Autodesk Inventor part; units mm, degrees
ref_plane "YZ Plane" through (0, 0, 0) normal (1, 0, 0) x (0, 1, 0)
ref_plane "XZ Plane" through (0, 0, 0) normal (0, 1, 0) x (-1, 0, 0)
ref_plane "XY Plane" through (0, 0, 0) normal (0, 0, 1) x (1, 0, 0)
sketch "スケッチ1" plane through (0, 0, 0) normal (0, 0, 1) x (1, 0, 0)
  line L0 (-22.9, 20) -> (-3.9468, 3.447)
  line L1 (3.9468, 3.447) -> (22.9, 20)
  line L2 (-22.9, 20) -> (22.9, 20)
  line L3 (0, 0) -> (0, 20) construction
  line L4 (-22.9, 23) -> (22.9, 23)
  line L5 (22.9, 23) -> (22.9, 20)
  line L6 (22.9, 20) -> (-22.9, 20)
  line L7 (-22.9, 20) -> (-22.9, 23)
  line L8 (0, -407.3642) -> (0, 141.394)
  line L9 (0, 0) -> (0, 23)
  arc A0 (-3.9468, 3.447) -> (3.9468, 3.447) centre (0, 7.9661) ccw
  line L10 (0, -328.9702) -> (-1095, -328.9702)
  line L11 (22.9, 23) -> (25.1, 23)
  line L12 (25.1, 23) -> (25.1, 20)
  line L13 (25.1, 20) -> (26.6, 20)
  line L14 (26.6, 20) -> (26.6, 26)
  line L15 (26.6, 26) -> (-26.6, 26)
  line L16 (-26.6, 26) -> (-26.6, 20)
  line L17 (-26.6, 20) -> (-25.1, 20)
  line L18 (-25.1, 20) -> (-25.1, 23)
  line L19 (-25.1, 23) -> (-22.9, 23)
  line L20 (-22.9, 23) -> (-22.9, 63)
  line L21 (-22.9, 63) -> (22.9, 63)
  line L22 (22.9, 63) -> (22.9, 23)
  point P0 (0, 1.9661)
  point P1 (0, 26)
  point P2 (0, 63)
  dimension "d0" = 45.8
  dimension "d1" = 20
  dimension "d3" = 3
  dimension "d5" = 6
  dimension "d6" = 1095
  dimension "d8" = 2.2
  dimension "d9" = 1.5
  dimension "d10" = 3
  dimension "d14" = 40
revolve "回転1" add sketch "スケッチ1" angle 360 about axis through (0, -10, 0) along (0, 1, 0) contours L8 L4 L5 L2 | L2 L1 A0 L8 | L8 L15 L22 L4 | L22 L15 L14 L13 L12 L11
properties part number "Camera_mirror"
Check sheet for the modelled part. Datum: model origin and axes. Units: mm. A direction names the side the tool comes from. Give positions to 0.01 mm unless a question says otherwise; leave off trailing zeros. Order: outer loops, then holes, each group sorted by start corner. A loop starts at its lowest first (then second) coordinate and runs counter-clockwise, first axis right, second up. Notation, with made-up numbers: M 62,-16.75 L 106,-16.75 A25 cw 106,8.25 Z; hole C 66.5,61.5 d10. An arc over 180 degrees is marked long. Answer in a Markdown table with one row per item. Add a question column.
Q1. Thickness scan on L1, parallel to Z at x = 0, y = 21.1; L2, parallel to Z at x = -17, y = 22. Record the ranges inside material, lowest first.
Q2. Sectioned sample at C-C, the plane z = 0. Record the boundary of the cut face in (x, y), and give its area (3 significant figures).
Q3. Sectioned sample at B-B, the plane x = 0. Record the boundary of the cut face in (y, z).
Q4. Sectioned sample at D-D, the plane y = 5. Record the boundary of the cut face in (x, z).
Q5. Sectioned sample at A-A, the plane y = 22. Record the boundary of the cut face in (x, z).
Q6. Access from +Z, -Z, +X, -X, +Y, -Y to the whole of each face (thin tool, end or side, straight path). Record for faces 4 (the flat face through (0, 26, 0)), 5 (the cylindrical face through (-4.964, 21.479, -22.355)).
Q7. Gauge pin test, flat ends, axial feed: pin 1 Ø2 at (y, z) = (10.5, -0.5) entering from -X; pin 2 Ø1.5 at (x, z) = (10.5, -4.5) entering from -Y; pin 3 Ø3 at (y, z) = (21, 15.5) entering from +X; pin 4 Ø1.5 at (y, z) = (5, 8) entering from +X. Record the tip position at first contact, or that the pin passes through.
Q8. Release check for a two-part mould opening along Z. For faces 1 (the flat face through (20.3, 23, 11)), 2 (the conical face through (-1.11, 4.48, 5.01)), 3 (the flat face through (20, 20, -16)) record: released by +Z, released by -Z, zero draft, split by the parting line, or undercut.
Verdict:
| question | item | result |
|---|---|---|
| 1 | L1 | -26.6 to -25.1, -22.9 to 22.9, 25.1 to 26.6 |
| 1 | L2 | -20.46 to -18.47, -15.34 to 15.34, 18.47 to 20.46 |
| 2 | outline | M -26.6,20 L -25.1,20 L -25.1,23 L -22.9,23 L -22.9,20 L -3.95,3.45 A6 ccw 3.95,3.45 L 22.9,20 L 22.9,23 L 25.1,23 L 25.1,20 L 26.6,20 L 26.6,26 L -26.6,26 Z |
| 2 | area | 758 mm² |
| 3 | outline | M 3.45,-3.95 L 20,-22.9 L 23,-22.9 L 23,-25.1 L 20,-25.1 L 20,-26.6 L 26,-26.6 L 26,26.6 L 20,26.6 L 20,25.1 L 23,25.1 L 23,22.9 L 20,22.9 L 3.45,3.95 A6 ccw Z |
| 4 | outline | C 0,0 d11.45 |
| 5 | outline | C 0,0 d53.2; C 0,0 d45.8; hole C 0,0 d50.2 |
| 6 | face 4 | +Z, -Z, +X, -X, +Y |
| 6 | face 5 | -Y |
| 7 | pin 1 | x = -13.16 |
| 7 | pin 2 | y = 9.32 |
| 7 | pin 3 | x = 22.62 |
| 7 | pin 4 | through |
| 8 | face 1 | undercut |
| 8 | face 2 | split by the parting line |
| 8 | face 3 | zero draft |
